Here's the drawing with two shaded views (mm, measured from the low corner). I have some questions. Give positions to 0.01 mm unless a question says otherwise; leave off trailing zeros. Loops run counter-clockwise (first coordinate to the right, second up) from the corner with the lowest first, then second, coordinate; pieces in that order, holes last. Notation, with made-up numbers: M 71,26.25 L 115,26.25 A26 cw 115,51.25 Z; hole C 21.25,50.25 d1. An arc over 180 degrees is marked long. Put each result on its own line as item: value. Start each with the question number.
1) Please list where these lines run through material, in increasing order: line 1 along Z through (x, y) = (10.16, 6.5) (1 decimal); line 2 along X through (y, z) = (13.5, 96) (1 decimal); line 3 along X through (y, z) = (2.5, 10.5). Write a range as from..to.
2) If we mould it in two halves opening along Z, with no side actions, what happens to the marked faces 1, 2 and 3? For each: +Z half, -Z half, draft (parallel to the pull), parting line (faces both ways), or undercut.
3) Imagine slicing it at C-C (x = 86.36). Write out the boundary of the cut face in (y, z) (1 decimal).
4) Imagine slicing it at B-B (z = 36). Write out the boundary of the cut face in (x, y), then the cut area to 3 significant figures.
5) Imagine slicing it at A-A (x = 10.16). Write out the boundary of the cut face in (y, z) (1 decimal).
6) Imagine slicing it at D-D (z = 93.5). Write out the boundary of the cut face in (x, y) (1 decimal), then the cut area to 3 significant figures.
7) For P1, Ø14, axis at x = 35.56, z = 91.47, coming from the -Y side, with a flat end and sliding along its axis, tell me the tip position at first contact or that it passes through.
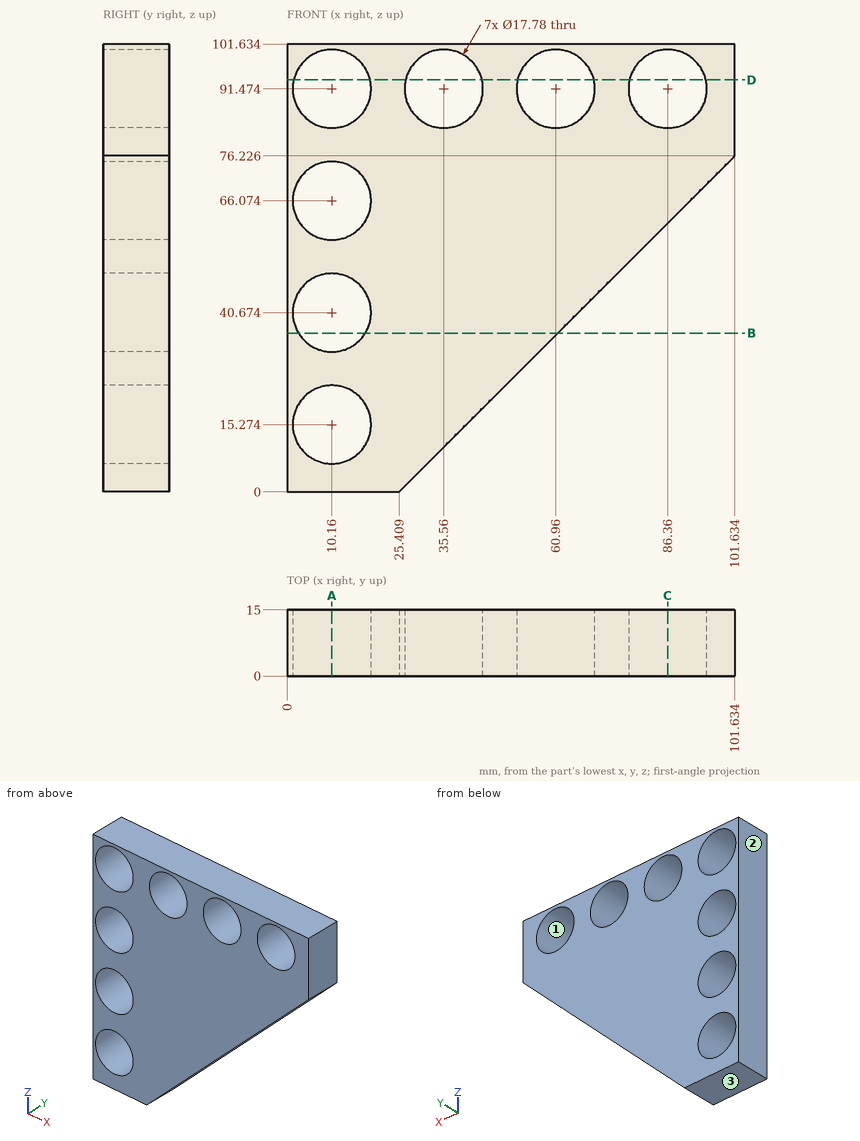
Recorded:
1. line 1: 0..6.4, 24.2..31.8, 49.6..57.2, 75..82.6, 100.4..101.6
1. line 2: 0..2.5, 17.8..27.9, 43.2..53.3, 68.6..78.7, 94..101.6
1. line 3: 0..2.66, 17.66..35.91
2. face 1: undercut
2. face 2: draft
2. face 3: -Z half
3. outline: M 0,61 L 15,61 L 15,82.6 L 0,82.6 Z; M 0,100.4 L 15,100.4 L 15,101.6 L 0,101.6 Z
4. outline: M 0,0 L 2.6,0 L 2.6,15 L 0,15 Z; M 17.72,0 L 61.41,0 L 61.41,15 L 17.72,15 Z
4. area: 694 mm²
5. outline: M 0,0 L 15,0 L 15,6.4 L 0,6.4 Z; M 0,24.2 L 15,24.2 L 15,31.8 L 0,31.8 Z; M 0,49.6 L 15,49.6 L 15,57.2 L 0,57.2 Z; M 0,75 L 15,75 L 15,82.6 L 0,82.6 Z; M 0,100.4 L 15,100.4 L 15,101.6 L 0,101.6 Z
6. outline: M 0,0 L 1.5,0 L 1.5,15 L 0,15 Z; M 18.8,0 L 26.9,0 L 26.9,15 L 18.8,15 Z; M 44.2,0 L 52.3,0 L 52.3,15 L 44.2,15 Z; M 69.6,0 L 77.7,0 L 77.7,15 L 69.6,15 Z; M 95,0 L 101.6,0 L 101.6,15 L 95,15 Z
6. area: 486 mm²
7. P1: through
